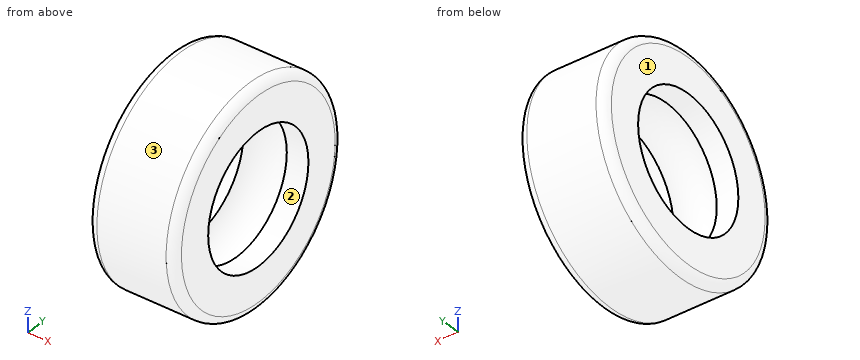
from build123d import *

# Parameters (mm, degrees)
FILLET1_R = 1


with BuildPart() as part:
    # Sketch1 → Revolve1 (revolve)
    with BuildSketch(Plane.XY, mode=Mode.PRIVATE) as revolve1_sk:
        with BuildLine():
            Line((2.5, 7.5), (5, 7.5))
            Line((5, 7.5), (5, 12.5))
            Line((5, 12.5), (-5, 12.5))
            Line((-5, 12.5), (-5, 7.5))
            Line((-5, 7.5), (-2.5, 7.5))
            ThreePointArc((-2.5, 7.5), (0, 10), (2.5, 7.5))
        make_face()
    revolve(revolve1_sk.sketch.rotate(Axis((0, 0, 0), (1, 0, 0)), 90), axis=Axis((0, 0, 0), (1, 0, 0)))

    # Fillet1
    fillet1_edges = [part.edges().sort_by_distance(p)[0] for p in [
        (-5, 0, -12.5),
        (5, 0, -12.5),
    ]]
    fillet(fillet1_edges, radius=FILLET1_R)


solid = part.part
Work out the finished part from the listing and answer in its coordinate system (mm). Face numbers are marked on the shaded views. Give positions to 0.01 mm unless a question says otherwise; leave off trailing zeros. Order: outer loops, then holes, each group sorted by start corner. A loop starts at its lowest first (then second) coordinate and runs counter-clockwise, first axis right, second up. Notation, with made-up numbers: (6.25, 18.25) -> (55.25, 18.25) arc R17 cw to (55.25, 36.25) -> close; hole circle Ø10 at (13.25, 16.25). An arc over 180 degrees is marked (long way). Answer as a JSON object with one key per item and string values. Group by question number.
1. The mould has two halves that part along Y. Classify the marked faces 1, 2 and 3: released by +Y, released by -Y, zero draft, split by the parting line, or undercut.
2. Flat-ended cylindrical pins translate along their axes: pin 1 Ø1 at (y, z) = (5.5, 4) entering from +X (3 decimals); pin 2 Ø1.5 at (x, y) = (0.5, 6) entering from +Z. Find the tip coordinate at first contact, or state that the pin passes through.
3. Section A-A on z = 0 is taken. Determine the outline of the cut face in (x, y).
4. Section C-C on x = -2 is taken. Determine the outline of the cut face in (y, z), plus the area to 3 significant figures.
5. Section D-D on x = 0 is taken. Determine the outline of the cut face in (y, z), plus the area to 3 significant figures.
6. Consider line 1 along Y through (x, z) = (3.3, 0); line 2 along X through (y, z) = (-9.5, 0); line 3 along Y through (x, z) = (0, -4.75). Determine where each line is inside the solid, lowest interval first. Write a range as [from, to].
Result sheet:
{
 "1": {"face 1": "zero draft", "face 2": "undercut", "face 3": "split by the parting line"},
 "2": {"pin 1": "passes through", "pin 2": "stops at z = 11.34"},
 "3": {"outline": "(-5, -11.5) arc R1 ccw to (-4, -12.5) -> (4, -12.5) arc R1 ccw to (5, -11.5) -> (5, -7.5) -> (2.5, -7.5) arc R2.5 cw to (-2.5, -7.5) -> (-5, -7.5) -> close; (-5, 7.5) -> (-2.5, 7.5) arc R2.5 cw to (2.5, 7.5) -> (5, 7.5) -> (5, 11.5) arc R1 ccw to (4, 12.5) -> (-4, 12.5) arc R1 ccw to (-5, 11.5) -> close"},
 "4": {"outline": "circle Ø25 at (0, 0); hole circle Ø18 at (0, 0)", "area": "236 mm^2"},
 "5": {"outline": "circle Ø25 at (0, 0); hole circle Ø20 at (0, 0)", "area": "177 mm^2"},
 "6": {"line 1": "y = [-12.5, -7.5], [7.5, 12.5]", "line 2": "x = [-5, -1.5], [1.5, 5]", "line 3": "y = [-11.56, -8.8], [8.8, 11.56]"}
}
